Here's how the part is built. I have some questions about the finished solid (model axes, mm). A direction names the side the tool comes from. Round coordinates to 2 decimals unless told otherwise and drop trailing zeros. Write each loop counter-clockwise with the first axis right and the second up, starting at its lowest first coordinate (ties: lowest second). Pieces come first, ordered by that corner, then holes. Notation, with made-up numbers: (64, 62) -> (79, 62) arc R25 ccw to (79, 95) -> close; hole circle Ø6 at (-37, 46.5). An arc over 180 degrees is marked (long way). Answer as CSV lines item,"result".
from build123d import *

# Parameters (mm, degrees)
F1_DEPTH = 2
F2_R     = 1.5
F3_DEPTH = 40
F4_SIZE  = 0.5


with BuildPart() as f1:
    # F0 (on Right) → F1 (new body)
    with BuildSketch(Plane.YZ):
        Polygon((1.587713, 2.75), (-1.587713, 2.75), (-3.175426, 0), (-1.587713, -2.75), (1.587713, -2.75), (3.175426, 0), align=None)
    extrude(amount=F1_DEPTH)

    # F2 (on Right) → F3 (join)
    with BuildSketch(Plane.YZ):
        Circle(F2_R)
    extrude(amount=-F3_DEPTH)

    # F4
    f4_edges = [f1.edges().sort_by_distance(p)[0] for p in [
        (-40, -1.5, 0),
    ]]
    chamfer(f4_edges, length=F4_SIZE)


solid = f1.part
Item 1: Suppose I cut it at C-C, the plane y = -2. List the corners of the cut face in (x, z) for me.
Results found:
outline,"(0, -2.04) -> (2, -2.04) -> (2, 2.04) -> (0, 2.04) -> close"
Item 2: Suppose I cut it at D-D, the plane y = 2.25. List the corners of the cut face in (x, z) for me, then the cut area to 3 significant figures.
Results found:
outline,"(0, -1.6) -> (2, -1.6) -> (2, 1.6) -> (0, 1.6) -> close"
area,"6.41 mm²"
Item 3: Suppose I cut it at A-A, the plane y = 0. List the corners of the cut face in (x, z) for me, then the cut area to 3 significant figures.
Results found:
outline,"(-40, -1) -> (-39.5, -1.5) -> (0, -1.5) -> (0, -2.75) -> (2, -2.75) -> (2, 2.75) -> (0, 2.75) -> (0, 1.5) -> (-39.5, 1.5) -> (-40, 1) -> close"
area,"131 mm²"
Item 4: Suppose I cut it at B-B, the plane x = -25.5. List the corners of the cut face in (y, z) for me, then the cut area to 3 significant figures.
Results found:
outline,"circle Ø3 at (0, 0)"
area,"7.07 mm²"
Item 5: For faces 1 (the flat face through (0.99, 2.39, 1.36)), 2 (the cylindrical face through (-19.47, -1.5, 0.07)), which set-ups out of +Z, -Z, +X, -X, +Y, -Y let a thin tool reach every point of the face, with its end or its side?
Results found:
face 1,"+Z, +X, -X, +Y"
face 2,"-X"
Item 6: I need wall thicknesses on L1, parallel to Y at x = -34.5, z = -0.15; L2, parallel to X at y = 2.5, z = 0.3; L3, parallel to Z at x = -22, y = 0. Which ranges of each line are inside material? Lowest first, please.
Results found:
L1,"y = -1.49 to 1.49"
L2,"x = 0 to 2"
L3,"z = -1.5 to 1.5"
Item 7: Will these pins go through, and if not, where does the flat tip stop? pin 1 (1.5 mm diameter, centred on x = -6.5, z = 0, fed in from -Y); pin 2 (3 mm diameter, centred on x = -30, y = 0, fed in from -Z).
Results found:
pin 1,"stops at y = -1.5"
pin 2,"stops at z = -1.5"
